from build123d import *

# Parameters (mm, degrees)
SKETCH_1_W      = 200
SKETCH_1_H      = 150
SKETCH_1_R      = 35
EXTRUDE_1_DEPTH = 18
FILLET_1_R      = 10


with BuildPart() as part:
    # 草图1 → 凸台-拉伸1 (new body)
    with BuildSketch(Plane(origin=(0, 0, 0), x_dir=(1, 0, 0), z_dir=(0, 1, 0))):
        Rectangle(SKETCH_1_W, SKETCH_1_H)
        with Locations(Location((40, 0, 0), (0, 0, 270))):
            Circle(SKETCH_1_R, mode=Mode.SUBTRACT)
    extrude(amount=EXTRUDE_1_DEPTH)

    # 圆角1
    fillet_1_edges = [part.edges().sort_by_distance(p)[0] for p in [
        (-100, 9, -75),
        (100, 9, -75),
        (100, 9, 75),
        (-100, 9, 75),
    ]]
    fillet(fillet_1_edges, radius=FILLET_1_R)


solid = part.part
For this review, take the finished solid that the model builds, in its own axes (mm). Round coordinates to 2 decimals unless told otherwise and drop trailing zeros. Order: outer loops, then holes, each group sorted by start corner. A loop starts at its lowest first (then second) coordinate and runs counter-clockwise, first axis right, second up. Notation, with made-up numbers: M 10.5,37 L 58.5,37 A16 cw 58.5,55 Z; hole C -4,55.5 d11. An arc over 180 degrees is marked long. Use a Markdown table: item, result. Add a question column.
Item 1: Add section B-B, the plane z = 0. Give the boundary of the cut face in (x, y).
Item 2: Mouldability with a two-part tool opening along X and no side actions: class faces 1 (the cylindrical face through (-97.15, 9.13, 71.99)), 2 (the cylindrical face through (74.7, 8.87, -4.56)), 3 (the cylindrical face through (96.99, 9.13, -72.15)), 4 (the flat face through (-1, 9, 75)) as released by +X, released by -X, zero draft, split by the parting line, or undercut.
Item 3: Add section A-A, the plane x = 40. Give the boundary of the cut face in (y, z).
Item 4: To check wall thickness, follow line 1 along X through (y, z) = (4.25, 0); line 2 along X through (y, z) = (13.75, 29); line 3 along Z through (x, y) = (70, 14.25). State the ranges of each line that lie inside material, in increasing order.
Item 5: Add section C-C, the plane y = 3.25. Give the boundary of the cut face in (x, z), then the cut area to 3 significant figures.
Geometry results:
| question | item | result |
|---|---|---|
| 1 | outline | M -100,0 L 5,0 L 5,18 L -100,18 Z; M 75,0 L 100,0 L 100,18 L 75,18 Z |
| 2 | face 1 | released by -X |
| 2 | face 2 | undercut |
| 2 | face 3 | released by +X |
| 2 | face 4 | zero draft |
| 3 | outline | M 0,-75 L 18,-75 L 18,-35 L 0,-35 Z; M 0,35 L 18,35 L 18,75 L 0,75 Z |
| 4 | line 1 | x = -100 to 5, 75 to 100 |
| 4 | line 2 | x = -100 to 20.4, 59.6 to 100 |
| 4 | line 3 | z = -75 to -18.03, 18.03 to 75 |
| 5 | outline | M -100,-65 A10 ccw -90,-75 L 90,-75 A10 ccw 100,-65 L 100,65 A10 ccw 90,75 L -90,75 A10 ccw -100,65 Z; hole C 40,0 d70 |
| 5 | area | 26,100 mm² |
